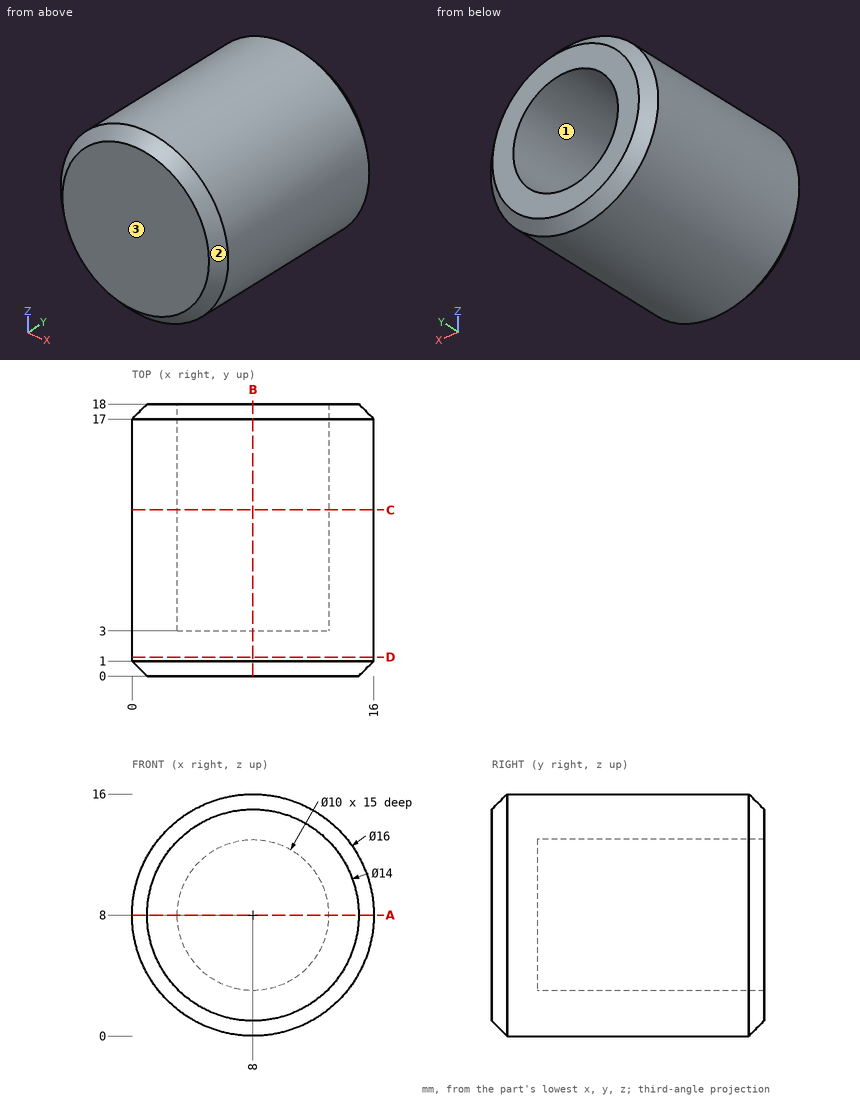
For this review, use the dimensioned drawing (mm, ordinates from the lowest corner) and the shaded views. Round coordinates to 2 decimals unless told otherwise and drop trailing zeros. Write each loop counter-clockwise with the first axis right and the second up, starting at its lowest first coordinate (ties: lowest second). Pieces come first, ordered by that corner, then holes. Notation, with made-up numbers: M 53.5,40 L 106.5,40 A32 ccw 106.5,75 Z; hole C 23.25,57.5 d9. An arc over 180 degrees is marked long. Answer as CSV lines item,"result". Start each with the question number.
Q1. Wall thickness on line 1 along Z through (x, y) = (8, 6.5); line 2 along Y through (x, z) = (9.25, 5); line 3 along X through (y, z) = (12, 12): over which ranges is each line inside the solid? List them lowest first.
Q2. Consider section B-B, the plane x = 8. Give the boundary of the cut face in (y, z), then the cut area to 3 significant figures.
Q3. Consider section A-A, the plane z = 8. Give the boundary of the cut face in (x, y).
Q4. Consider section D-D, the plane y = 1.25. Give the boundary of the cut face in (x, z), then the cut area to 3 significant figures.
Q5. The part is to be moulded in two halves that separate along X. For the marked faces 1, 2 and 3, say which applies: +X half, -X half, draft (parallel to the pull), parting line (faces both ways), or undercut.
Q6. Consider section C-C, the plane y = 11. Give the boundary of the cut face in (x, z), then the cut area to 3 significant figures.
Q7. Clearance check with flat-ended pins moving along their axes: P1, Ø8, axis at x = 8, z = 8, coming from the +Y side; P2, Ø2, axis at x = 3.5, y = 12, coming from the +Z side; P3, Ø5, axis at x = 9, y = 13, coming from the +Z side. State where each tip first meets the part, or that it passes through.
Result set:
1,line 1,"z = 0 to 3, 13 to 16"
1,line 2,"y = 0 to 3"
1,line 3,"x = 1.07 to 5, 11 to 14.93"
2,outline,"M 0,1 L 1,0 L 17,0 L 18,1 L 18,3 L 3,3 L 3,13 L 18,13 L 18,15 L 17,16 L 1,16 L 0,15 Z"
2,area,"136 mm²"
3,outline,"M 0,1 L 1,0 L 15,0 L 16,1 L 16,17 L 15,18 L 13,18 L 13,3 L 3,3 L 3,18 L 1,18 L 0,17 Z"
4,outline,"C 8,8 d16"
4,area,"201 mm²"
5,face 1,"undercut"
5,face 2,"parting line"
5,face 3,"draft"
6,outline,"C 8,8 d16; hole C 8,8 d10"
6,area,"123 mm²"
7,P1,"stops at y = 3"
7,P2,"stops at z = 15.19"
7,P3,"stops at z = 16"
